Solid Edge part; units mm, degrees
sketch "Sketch1" plane through (0, 0, 0) normal (0, 0, 1) x (1, 0, 0)
  line L0 (15.5, -13.4968) -> (13.5, -13.5001)
  line L1 (13.5, -13.5001) -> (13.5, 13.4999)
  line L2 (13.5, 13.4999) -> (-13.5, 13.4999)
  line L3 (-13.5, 13.4999) -> (-13.5, -13.5001)
  line L4 (-13.5, -13.5001) -> (-15.5, -13.5001)
  line L5 (-15.5, -13.5001) -> (-15.5, 15.4999)
  line L6 (-15.5, 15.4999) -> (15.5, 15.4999)
  line L7 (15.5, 15.4999) -> (15.5, -13.5001)
extrude "Protrusion1" add sketch "Sketch1" along normal blind 4
sketch "Sketch2" plane through (-13.5, -0.0001, 2) normal (1, 0, 0) x (0, 1, 0)
  line L0 (-2.4979, 1.9971) -> (-2.4979, 0.9971)
  line L1 (-2.4979, 0.9971) -> (2.5021, 0.9971)
  line L2 (2.5021, 0.9971) -> (2.5021, 1.9971)
  line L3 (2.5021, 1.9971) -> (-2.4979, 1.9971)
extrude "ExtrudedProtrusion_10" add sketch "Sketch2" along normal blind 2.5
sketch "Sketch3" plane through (13.5, -0.0001, 2) normal (-1, 0, 0) x (0, -1, 0)
  line L0 (2.5034, 2) -> (-2.4966, 2)
  line L1 (-2.4966, 2) -> (-2.4966, 1.0032)
  line L2 (-2.4966, 1.0032) -> (2.5034, 1.0032)
  line L3 (2.5034, 1.0032) -> (2.5034, 2)
extrude "ExtrudedProtrusion_11" add sketch "Sketch3" along normal blind 2.5
Input: part model. Units: mm. Frame: model coordinates. A direction names the side the tool comes from. Round coordinates to 2 decimals unless told otherwise and drop trailing zeros. Order: outer loops, then holes, each group sorted by start corner. A loop starts at its lowest first (then second) coordinate and runs counter-clockwise, first axis right, second up. Notation, with made-up numbers: (32, 42.5) - (37, 42.5) arc R34 ccw to (37, 77.5) - close; hole circle Ø5 at (64, -6). An arc over 180 degrees is marked (long way). Use a Markdown table: item, result.
1. Access query for faces 1 (the face through (-12, 0, 2.997)), 2 (the face through (15.5, 1, 2)), 3 (the face through (12.3, 2.496, 3.5)), 4 (the face through (-12.3, -2.498, 3.5)). Directions: +Z, -Z, +X, -X, +Y, -Y. A direction counts if a zero-diameter tool reaches every point of the face in a straight line with its end or side. Return the directions, or none.
Evaluation:
| item | result |
|---|---|
| face 1 | -Z, -Y |
| face 2 | +Z, -Z, +X, +Y, -Y |
| face 3 | +Z, -Z |
| face 4 | +Z, -Z, -Y |
2. Material intervals for probe 1 along X at (y, z) = (0.5, 2.6); probe 2 along Y at (x, z) = (12, 3.35); probe 3 along Y at (x, z) = (0.5, 1.4), sorted ascending.
Evaluation:
| item | result |
|---|---|
| probe 1 | -15.5 to -13.5, 13.5 to 15.5 |
| probe 2 | -2.5 to 2.5, 13.5 to 15.5 |
| probe 3 | 13.5 to 15.5 |
3. Section A-A on y = -3. Return the cut outline in (x, z).
Evaluation:
| item | result |
|---|---|
| outline | (-15.5, 0) - (-13.5, 0) - (-13.5, 4) - (-15.5, 4) - close; (13.5, 0) - (15.5, 0) - (15.5, 4) - (13.5, 4) - close |
4. Mould query, pull axis X, two halves, no side actions, for faces 5 (the face through (-13.5, 0, 2)), 6 (the face through (2, 14, 0)), 7 (the face through (-15.5, 1, 2)). Classes: +X half, -X half, draft (parallel to the pull), parting line (faces both ways), or undercut.
Evaluation:
| item | result |
|---|---|
| face 5 | undercut |
| face 6 | draft |
| face 7 | -X half |
5. First-contact query: pin 1 (1.5 mm diameter, centred on x = 10, z = 1.5, fed in from -Y); pin 2 (12 mm diameter, centred on x = 7, y = -10.5, fed in from +Z); pin 3 (1.2 mm diameter, centred on x = 12, y = 0.5, fed in from -Z); pin 4 (0.5 mm diameter, centred on x = 12, z = 3.5, fed in from -Y). Flat tips, straight axial feed; report the tip coordinate or a pass-through.
Evaluation:
| item | result |
|---|---|
| pin 1 | y = 13.5 |
| pin 2 | through |
| pin 3 | z = 3 |
| pin 4 | y = -2.5 |
6. Section D-D on x = 1.5. Return the cut outline in (y, z).
Evaluation:
| item | result |
|---|---|
| outline | (13.5, 0) - (15.5, 0) - (15.5, 4) - (13.5, 4) - close |
7. Section B-B on x = 13. Return the cut outline in (y, z).
Evaluation:
| item | result |
|---|---|
| outline | (-2.5, 3) - (2.5, 3) - (2.5, 4) - (-2.5, 4) - close; (13.5, 0) - (15.5, 0) - (15.5, 4) - (13.5, 4) - close |
8. Section C-C on z = 2.6. Return the cut outline in (x, y).
Evaluation:
| item | result |
|---|---|
| outline | (-15.5, -13.5) - (-13.5, -13.5) - (-13.5, 13.5) - (13.5, 13.5) - (13.5, -13.5) - (15.5, -13.5) - (15.5, 15.5) - (-15.5, 15.5) - close |
